Design review of the part shown in the three views and the two pictorial views. Dimensions are in mm from the part's minimum x, y and z. A direction names the side the tool comes from. Coordinates: 2 decimals unless noted, no trailing zeros. Loops run counter-clockwise (first coordinate to the right, second up) from the corner with the lowest first, then second, coordinate; pieces in that order, holes last.
Q1. Add section D-D on z = 8. Give the boundary of the cut face in (x, y) (1 decimal).
Q2. Add section B-B on z = 20. Give the boundary of the cut face in (x, y).
Q3. For P1, Ø11.5, axis at x = 20, y = 11.5, coming from the -Z side; P2, Ø2, axis at x = 18.5, y = 39, coming from the -Z side; P3, Ø10, axis at x = 9.5, y = 33.5, coming from the +Z side, all flat-tipped, find the tip position at first contact; note any pin that passes through.
Q4. Wall thickness on probe 1 along Y at (x, z) = (28.5, 32); probe 2 along Z at (x, y) = (25, 34); probe 3 along Y at (x, z) = (45.5, 33.5): over which ranges is each line inside the solid? List them lowest first.
Q5. Add section A-A on x = 19.5. Give the boundary of the cut face in (y, z), and give its area (3 significant figures).
Q6. Machinability: for the marked faces 1, 2, 3 and 4, which of the approach directions +Z, -Z, +X, -X, +Y, -Y give a long, thin tool a straight path to every point of the face, cutting with its end or side? Answer none if there is none.
Q7. Add section C-C on y = 10. Give the boundary of the cut face in (x, z).
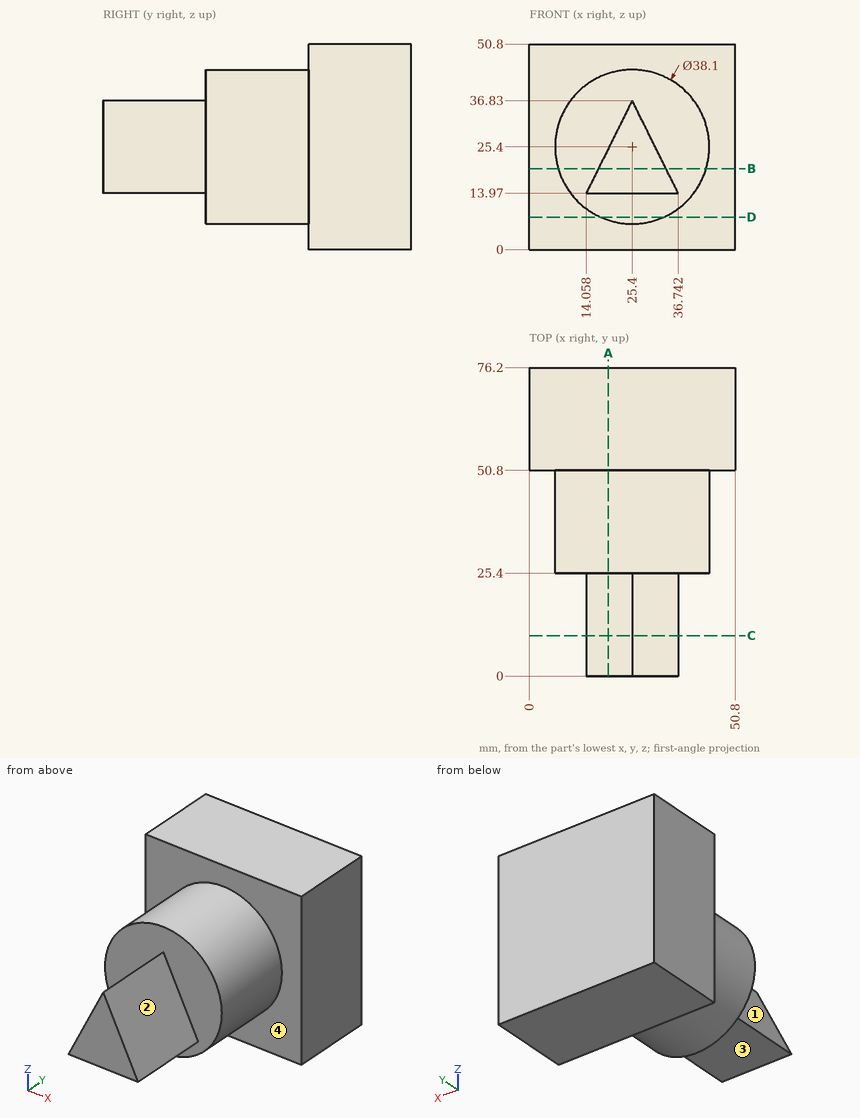
Entries:
1. outline: (0, 50.8) - (17.6, 50.8) - (17.6, 25.4) - (33.2, 25.4) - (33.2, 50.8) - (50.8, 50.8) - (50.8, 76.2) - (0, 76.2) - close
2. outline: (0, 50.8) - (7.13, 50.8) - (7.13, 25.4) - (17.05, 25.4) - (17.05, 0) - (33.75, 0) - (33.75, 25.4) - (43.67, 25.4) - (43.67, 50.8) - (50.8, 50.8) - (50.8, 76.2) - (0, 76.2) - close
3. P1: stops at z = 13.97
3. P2: stops at z = 7.29
3. P3: stops at z = 41.02
4. probe 1: y = 25.4 to 76.2
4. probe 2: z = 6.35 to 44.45
4. probe 3: y = 50.8 to 76.2
5. outline: (0, 13.97) - (25.4, 13.97) - (25.4, 7.29) - (50.8, 7.29) - (50.8, 0) - (76.2, 0) - (76.2, 50.8) - (50.8, 50.8) - (50.8, 43.51) - (25.4, 43.51) - (25.4, 24.94) - (0, 24.94) - close
5. area: 2,490 mm2
6. face 1: +Z, -X, -Y
6. face 2: +Z, +X, -Y
6. face 3: -Z, +X, -X, -Y
6. face 4: -Y
7. outline: (14.06, 13.97) - (36.74, 13.97) - (25.4, 36.83) - close
